Job drawing, mm, ordinate dimensions from the low corner. One solid piece. A direction names the side the tool comes from. Give positions to 0.01 mm unless a question says otherwise; leave off trailing zeros. Loops run counter-clockwise (first coordinate to the right, second up) from the corner with the lowest first, then second, coordinate; pieces in that order, holes last.
Item 1: Saw through at C-C on y = 14.25. Give the cut face in (x, z), plus the area to 3 significant figures.
Item 2: Saw through at A-A on y = 1.75. Give the cut face in (x, z), plus the area to 3 significant figures.
Item 3: Saw through at B-B on x = 14. Give the cut face in (y, z).
Item 4: Which spindle directions (+Z, -Z, +X, -X, +Y, -Y) get a long thin tool onto all of the face, cutting with end or side? Do the marked faces 5, 6 and 7. Say none if no direction does.
Item 5: Saw through at D-D on z = 3.9. Give the cut face in (x, y).
Item 6: Probe probe 1 along X at (y, z) = (4, 0.6) (1 decimal); probe 2 along X at (y, z) = (2, 0.75); probe 3 along X at (y, z) = (14, 3.45) (1 decimal). List the from-to ranges inside material, lowest first.
Item 7: Drop flat-ended pins along their axis: P1, Ø1.8, axis at y = 14.5, z = 3, coming from the -X side; P2, Ø3, axis at x = 25.5, z = 3.5, coming from the +Y side; P3, Ø1.5, axis at y = 22, z = 2, coming from the -X side (1 decimal); P4, Ø2, axis at x = 25.5, y = 5.5, coming from the +Z side. Give the stop position or say it passes through.
Item 8: Mould opens along Y. For the marked faces 1, 2, 3 and 4 say: released by +Y, released by -Y, zero draft, split by the parting line, or undercut.
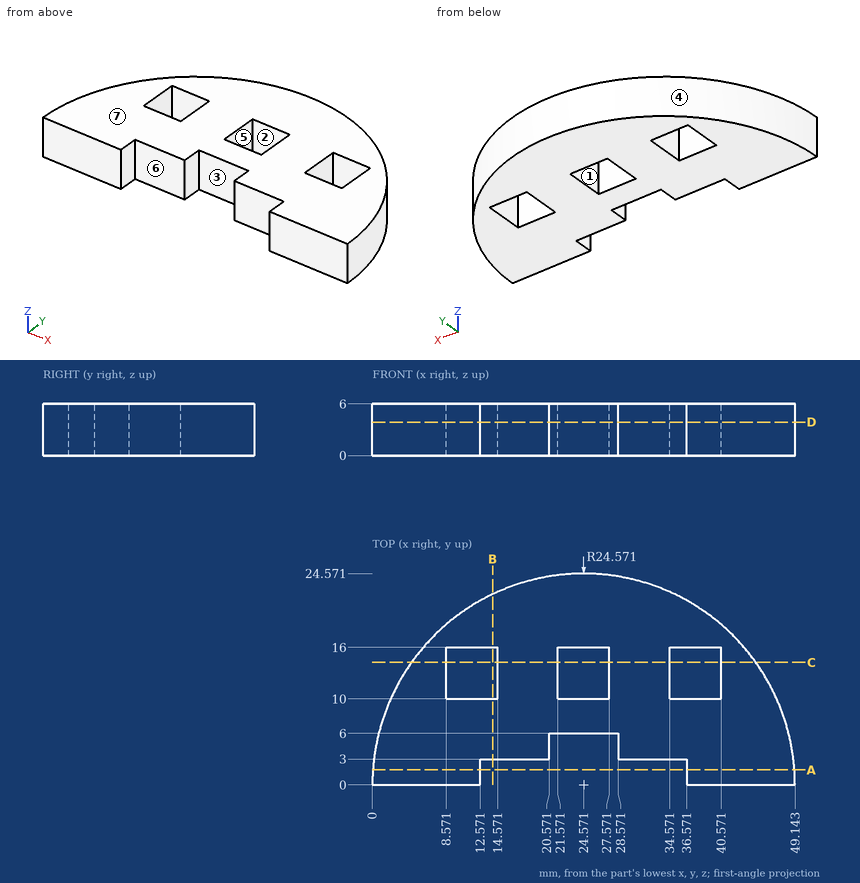
Results below:
1. outline: (4.55, 0) - (8.57, 0) - (8.57, 6) - (4.55, 6) - close; (14.57, 0) - (21.57, 0) - (21.57, 6) - (14.57, 6) - close; (27.57, 0) - (34.57, 0) - (34.57, 6) - (27.57, 6) - close; (40.57, 0) - (44.59, 0) - (44.59, 6) - (40.57, 6) - close
1. area: 132 mm2
2. outline: (0.06, 0) - (12.57, 0) - (12.57, 6) - (0.06, 6) - close; (36.57, 0) - (49.08, 0) - (49.08, 6) - (36.57, 6) - close
2. area: 150 mm2
3. outline: (3, 0) - (10, 0) - (10, 6) - (3, 6) - close; (16, 0) - (22.18, 0) - (22.18, 6) - (16, 6) - close
4. face 5: +Z, -Z
4. face 6: +Z, -Z, -Y
4. face 7: +Z, +X, -X, +Y, -Y
5. outline: (0, 0) - (12.57, 0) - (12.57, 3) - (20.57, 3) - (20.57, 6) - (28.57, 6) - (28.57, 3) - (36.57, 3) - (36.57, 0) - (49.14, 0) arc R24.57 ccw to start; hole (8.57, 10) - (14.57, 10) - (14.57, 16) - (8.57, 16) - close; hole (21.57, 10) - (27.57, 10) - (27.57, 16) - (21.57, 16) - close; hole (34.57, 10) - (40.57, 10) - (40.57, 16) - (34.57, 16) - close
6. probe 1: x = 0.3 to 20.6, 28.6 to 48.8
6. probe 2: x = 0.08 to 12.57, 36.57 to 49.06
6. probe 3: x = 4.4 to 8.6, 14.6 to 21.6, 27.6 to 34.6, 40.6 to 44.8
7. P1: stops at x = 4.11
7. P2: stops at y = 24.57
7. P3: stops at x = 12.2
7. P4: stops at z = 6
8. face 1: undercut
8. face 2: undercut
8. face 3: released by -Y
8. face 4: released by +Y
